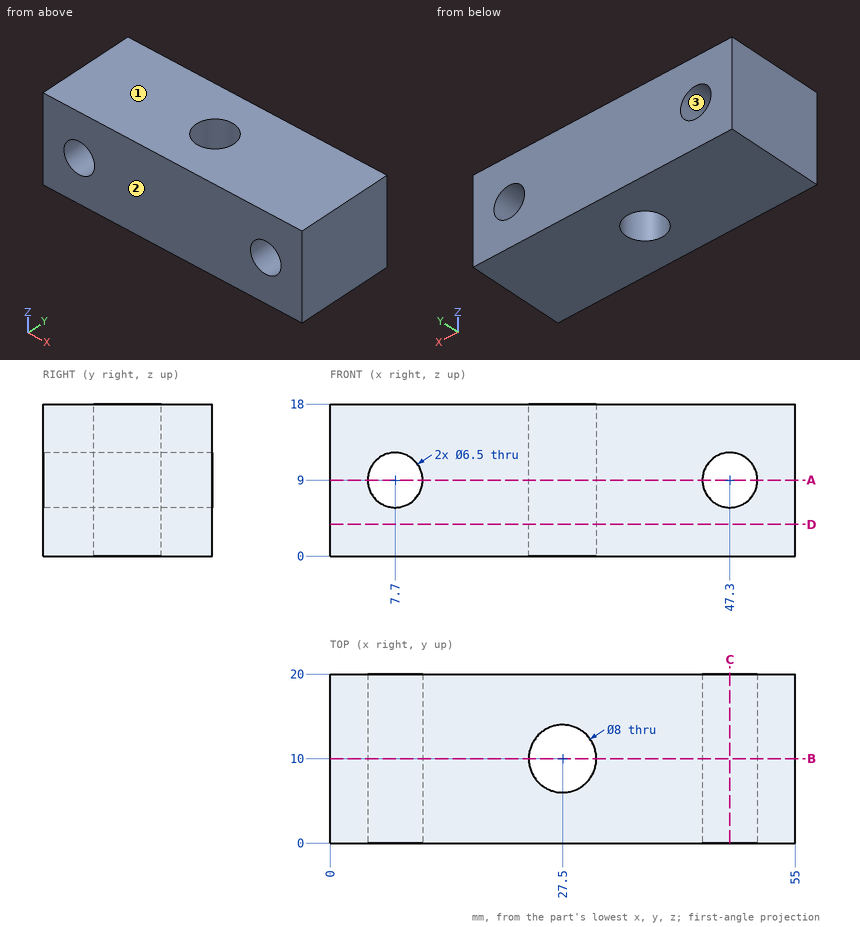
Input: dimensioned drawing with shaded views. Units: mm. Origin: part minimum x, y, z. Round coordinates to 2 decimals unless told otherwise and drop trailing zeros. Order: outer loops, then holes, each group sorted by start corner. A loop starts at its lowest first (then second) coordinate and runs counter-clockwise, first axis right, second up. Notation, with made-up numbers: (17.25, 79.5) - (26.25, 79.5) arc R22 ccw to (26.25, 116.5) - close; hole circle Ø4 at (9, 89). An arc over 180 degrees is marked (long way). Answer as a JSON object with one key per item and string values. Group by question number.
(1) Material intervals for probe 1 along X at (y, z) = (9.75, 9); probe 2 along Z at (x, y) = (7.7, 14.25); probe 3 along Y at (x, z) = (27.5, 6.5), sorted ascending. Write a range as from..to.
(2) Pin query (flat end, axial travel): P1, Ø3, axis at x = 38.5, y = 8.5, coming from the -Z side. Return the tip coordinate at first contact, or that it passes through.
(3) Cut plane C-C (x = 47.3). Return loops of the section in (y, z), then the cut area to 3 significant figures.
(4) Cut plane B-B (y = 10). Return loops of the section in (x, z), then the cut area to 3 significant figures.
(5) Draft query along Z for the marked faces 1, 2 and 3. Return one class per face: released by +Z, released by -Z, zero draft, split by the parting line, or undercut.
(6) Cut plane D-D (z = 3.75). Return loops of the section in (x, y), then the cut area to 3 significant figures.
(7) Cut plane A-A (z = 9). Return loops of the section in (x, y), then the cut area to 3 significant figures.
Here are the results:
{
 "1": {"probe 1": "x = 0..4.45, 10.95..23.51, 31.49..44.05, 50.55..55", "probe 2": "z = 0..5.75, 12.25..18", "probe 3": "y = 0..6, 14..20"},
 "2": {"P1": "stops at z = 0"},
 "3": {"outline": "(0, 0) - (20, 0) - (20, 5.75) - (0, 5.75) - close; (0, 12.25) - (20, 12.25) - (20, 18) - (0, 18) - close", "area": "230 mm^2"},
 "4": {"outline": "(0, 0) - (23.5, 0) - (23.5, 18) - (0, 18) - close; (31.5, 0) - (55, 0) - (55, 18) - (31.5, 18) - close; hole circle Ø6.5 at (7.7, 9); hole circle Ø6.5 at (47.3, 9)", "area": "780 mm^2"},
 "5": {"face 1": "released by +Z", "face 2": "zero draft", "face 3": "undercut"},
 "6": {"outline": "(0, 0) - (55, 0) - (55, 20) - (0, 20) - close; hole circle Ø8 at (27.5, 10)", "area": "1,050 mm^2"},
 "7": {"outline": "(0, 0) - (4.45, 0) - (4.45, 20) - (0, 20) - close; (10.95, 0) - (44.05, 0) - (44.05, 20) - (10.95, 20) - close; (50.55, 0) - (55, 0) - (55, 20) - (50.55, 20) - close; hole circle Ø8 at (27.5, 10)", "area": "790 mm^2"}
}
